Source: CAD feature listing. Evaluate the final solid. Frame: model axes, mm. A direction names the side the tool comes from. Round coordinates to 2 decimals unless told otherwise and drop trailing zeros. Loops run counter-clockwise (first coordinate to the right, second up) from the corner with the lowest first, then second, coordinate; pieces in that order, holes last. Notation, with made-up numbers: M 19,47.25 L 48,47.25 A28 cw 48,84.25 Z; hole C -39.5,-7 d9. An arc over 180 degrees is marked long. Answer as a JSON object with one key per item and string values.
Autodesk Inventor part; units mm, degrees
ref_plane "YZ Plane" through (0, 0, 0) normal (1, 0, 0) x (0, 1, 0)
ref_plane "XZ Plane" through (0, 0, 0) normal (0, 1, 0) x (-1, 0, 0)
ref_plane "XY Plane" through (0, 0, 0) normal (0, 0, 1) x (1, 0, 0)
sketch "Sketch1" plane through (0, 0, 0) normal (0, 1, 0) x (-1, 0, 0)
  line L0 (0, 0) -> (27, 0)
  line L1 (27, 0) -> (27, -65)
  line L2 (27, -65) -> (0, -65)
  line L3 (0, -65) -> (0, 0)
  dimension "d0" = 27
  dimension "d1" = 65
extrude "Extrusion1" add sketch "Sketch1" along normal blind 1
sketch "Sketch2" plane through (0, 1, 0) normal (0, 1, 0) x (1, 0, 0)
  line L0 (-27, 0) -> (0, 0)
  line L1 (0, 65) -> (-27, 65)
  line L2 (-13.5, 0) -> (-20, 0)
  line L3 (-20, 0) -> (-7, 0)
  line L4 (-7, 0) -> (-7, 65)
  line L5 (-20, 0) -> (-20, 65)
  line L6 (-7, 65) -> (-20, 65)
  dimension "d4" = 6.5
  dimension "d5" = 13
extrude "Extrusion2" add sketch "Sketch2" along normal blind 2
sketch "Sketch3" plane through (0, 3, 0) normal (0, 1, 0) x (1, 0, 0)
  line L0 (-7, 0) -> (-7, 65)
  line L1 (-7, 65) -> (-20, 65)
  line L2 (-7, 0) -> (-9, 0)
  line L3 (-9, 0) -> (-9, 65)
  line L4 (-9, 65) -> (-7, 65)
  line L5 (-7, 65) -> (-7, 0)
  point P0 (0, 0)
  dimension "d8" = 2
extrude "Extrusion3" add sketch "Sketch3" along normal blind 20
sketch "Sketch4" plane through (0, 23, 0) normal (0, 1, 0) x (1, 0, 0)
  line L0 (-20, 0) -> (-20, 65)
  line L1 (-7, 0) -> (-20, 0)
  line L2 (-20, 0) -> (-20, 65)
  line L3 (-20, 65) -> (-7, 65)
  line L4 (-7, 65) -> (-7, 0)
  point P0 (0, 0)
extrude "Extrusion4" add sketch "Sketch4" along normal blind 2
sketch "Sketch5" plane through (-7, 1, 0) normal (1, 0, 0) x (0, 0, -1)
  line L0 (65, 0) -> (65, 24)
  line L1 (0, 0) -> (0, 24)
  line L2 (0, 12) -> (65, 12)
  circle A0 centre (32.5, 12) radius 3
  point P0 (0, -1)
  dimension "d13" = 6
extrude "Extrusion5" cut sketch "Sketch5" against normal blind 2
properties part number "EE Track"
Item 1: Line query: probe 1 along Y at (x, z) = (-8.4, -32.5); probe 2 along Y at (x, z) = (-18.5, -13); probe 3 along Z at (x, y) = (-7.5, 13). Output: solid intervals per line, ascending. Write a range as from..to.
Answer sheet:
{"probe 1": "y = 0..10, 16..25", "probe 2": "y = 0..3, 23..25", "probe 3": "z = -65..-35.5, -29.5..0"}
Item 2: Section D-D on z = -6. Return the cut outline in (x, y).
Answer sheet:
{"outline": "M -27,0 L 0,0 L 0,1 L -7,1 L -7,25 L -20,25 L -20,23 L -9,23 L -9,3 L -20,3 L -20,1 L -27,1 Z"}
Item 3: Section C-C on x = -16. Return the cut outline in (y, z), then the cut area to 3 significant figures.
Answer sheet:
{"outline": "M 0,-65 L 3,-65 L 3,0 L 0,0 Z; M 23,-65 L 25,-65 L 25,0 L 23,0 Z", "area": "325 mm²"}
Item 4: Contact query for flat-ended pins moving along their axis: pin 1 Ø8 at (y, z) = (13, -32.5) entering from -X; pin 2 Ø7.5 at (x, z) = (-2, -23) entering from +Y; pin 3 Ø5 at (y, z) = (6, -50.5) entering from +X. Output: stop coordinate, or through.
Answer sheet:
{"pin 1": "stops at x = -9", "pin 2": "stops at y = 1", "pin 3": "stops at x = -7"}
Item 5: Pull-direction query (Y, two-part tool) for faces 4 (the cylindrical face through (-8, 13.1, -29.5)), 5 (the flat face through (-13, 0, -32)), 6 (the flat face through (-15, 3, -33)), 7 (the flat face through (-20, 24, -32)); classes: pulls with the +Y half, pulls with the -Y half, needs draft (parallel to the pull), parting line crosses it, or undercut.
Answer sheet:
{"face 4": "undercut", "face 5": "pulls with the -Y half", "face 6": "undercut", "face 7": "needs draft"}
Item 6: Access query for faces 1 (the flat face through (-9, 8, -32)), 2 (the flat face through (-3, 1, -32)), 3 (the flat face through (-20, 2, -32)). Directions: +Z, -Z, +X, -X, +Y, -Y. A direction counts if a zero-diameter tool reaches every point of the face in a straight line with its end or side. Return the directions, or none.
Answer sheet:
{"face 1": "+Z, -Z, -X", "face 2": "+Z, -Z, +X, +Y", "face 3": "+Z, -Z, -X, +Y"}
Item 7: Section B-B on z = -32.5. Return the cut outline in (x, y), then the cut area to 3 significant figures.
Answer sheet:
{"outline": "M -27,0 L 0,0 L 0,1 L -7,1 L -7,10 L -9,10 L -9,3 L -20,3 L -20,1 L -27,1 Z; M -20,23 L -9,23 L -9,16 L -7,16 L -7,25 L -20,25 Z", "area": "107 mm²"}
Item 8: Section A-A on y = 13. Return the cut outline in (x, z), then the cut area to 3 significant figures.
Answer sheet:
{"outline": "M -9,-65 L -7,-65 L -7,-35.5 L -9,-35.5 Z; M -9,-29.5 L -7,-29.5 L -7,0 L -9,0 Z", "area": "118 mm²"}
